```python
from build123d import *

# Parameters (mm, degrees)
SKETCH_1_W      = 292
SKETCH_1_H      = 160
SKETCH_1_R      = 1.5
SKETCH_1_W_2    = 60
SKETCH_1_H_2    = 80
EXTRUDE_1_DEPTH = 2


with BuildPart() as part:
    # 草图1 → 凸台-拉伸1 (new body)
    with BuildSketch(Plane(origin=(0, 0, 0), x_dir=(1, 0, 0), z_dir=(0, 1, 0))):
        with Locations((146, 80)):
            Rectangle(SKETCH_1_W, SKETCH_1_H)
        with Locations(Location((3, 140, 0), (0, 0, 270))):
            Circle(SKETCH_1_R, mode=Mode.SUBTRACT)
        with Locations(Location((3, 120, 0), (0, 0, 270))):
            Circle(SKETCH_1_R, mode=Mode.SUBTRACT)
        with Locations(Location((3, 40, 0), (0, 0, 270))):
            Circle(SKETCH_1_R, mode=Mode.SUBTRACT)
        with Locations(Location((3, 20, 0), (0, 0, 270))):
            Circle(SKETCH_1_R, mode=Mode.SUBTRACT)
        with Locations(Location((289, 20, 0), (0, 0, 90))):
            Circle(SKETCH_1_R, mode=Mode.SUBTRACT)
        with Locations(Location((289, 40, 0), (0, 0, 90))):
            Circle(SKETCH_1_R, mode=Mode.SUBTRACT)
        with Locations(Location((289, 120, 0), (0, 0, 90))):
            Circle(SKETCH_1_R, mode=Mode.SUBTRACT)
        with Locations(Location((289, 140, 0), (0, 0, 90))):
            Circle(SKETCH_1_R, mode=Mode.SUBTRACT)
        with Locations(Location((187, 120, 0), (0, 0, 270))):
            Circle(SKETCH_1_R, mode=Mode.SUBTRACT)
        with Locations(Location((262, 120, 0), (0, 0, 270))):
            Circle(SKETCH_1_R, mode=Mode.SUBTRACT)
        with Locations(Location((262, 98, 0), (0, 0, 270))):
            Circle(SKETCH_1_R, mode=Mode.SUBTRACT)
        with Locations(Location((187, 98, 0), (0, 0, 270))):
            Circle(SKETCH_1_R, mode=Mode.SUBTRACT)
        with Locations(Location((187, 105, 0), (0, 0, 270))):
            Circle(SKETCH_1_R, mode=Mode.SUBTRACT)
        with Locations(Location((262, 105, 0), (0, 0, 270))):
            Circle(SKETCH_1_R, mode=Mode.SUBTRACT)
        with Locations(Location((187, 83, 0), (0, 0, 270))):
            Circle(SKETCH_1_R, mode=Mode.SUBTRACT)
        with Locations(Location((262, 83, 0), (0, 0, 270))):
            Circle(SKETCH_1_R, mode=Mode.SUBTRACT)
        with Locations(Location((187, 90, 0), (0, 0, 270))):
            Circle(SKETCH_1_R, mode=Mode.SUBTRACT)
        with Locations(Location((262, 90, 0), (0, 0, 270))):
            Circle(SKETCH_1_R, mode=Mode.SUBTRACT)
        with Locations(Location((187, 68, 0), (0, 0, 270))):
            Circle(SKETCH_1_R, mode=Mode.SUBTRACT)
        with Locations(Location((262, 68, 0), (0, 0, 270))):
            Circle(SKETCH_1_R, mode=Mode.SUBTRACT)
        with Locations(Location((187, 75, 0), (0, 0, 270))):
            Circle(SKETCH_1_R, mode=Mode.SUBTRACT)
        with Locations(Location((262, 75, 0), (0, 0, 270))):
            Circle(SKETCH_1_R, mode=Mode.SUBTRACT)
        with Locations(Location((187, 53, 0), (0, 0, 270))):
            Circle(SKETCH_1_R, mode=Mode.SUBTRACT)
        with Locations(Location((262, 53, 0), (0, 0, 270))):
            Circle(SKETCH_1_R, mode=Mode.SUBTRACT)
        with Locations(Location((187, 60, 0), (0, 0, 270))):
            Circle(SKETCH_1_R, mode=Mode.SUBTRACT)
        with Locations(Location((262, 60, 0), (0, 0, 270))):
            Circle(SKETCH_1_R, mode=Mode.SUBTRACT)
        with Locations(Location((187, 38, 0), (0, 0, 270))):
            Circle(SKETCH_1_R, mode=Mode.SUBTRACT)
        with Locations(Location((262, 38, 0), (0, 0, 270))):
            Circle(SKETCH_1_R, mode=Mode.SUBTRACT)
        with Locations(Location((40, 145, 0), (0, 0, 270))):
            Circle(SKETCH_1_R, mode=Mode.SUBTRACT)
        with Locations(Location((80, 145, 0), (0, 0, 270))):
            Circle(SKETCH_1_R, mode=Mode.SUBTRACT)
        with Locations(Location((40, 15, 0), (0, 0, 270))):
            Circle(SKETCH_1_R, mode=Mode.SUBTRACT)
        with Locations(Location((80, 15, 0), (0, 0, 270))):
            Circle(SKETCH_1_R, mode=Mode.SUBTRACT)
        with Locations((60, 80)):
            Rectangle(SKETCH_1_W_2, SKETCH_1_H_2, mode=Mode.SUBTRACT)
        with BuildLine():
            Line((197, 124), (252, 124))
            ThreePointArc((252, 124), (256, 120), (252, 116))
            Line((252, 116), (197, 116))
            ThreePointArc((197, 116), (193, 120), (197, 124))
        make_face(mode=Mode.SUBTRACT)
        with BuildLine():
            Line((197, 101), (252, 101))
            ThreePointArc((252, 101), (256, 105), (252, 109))
            Line((252, 109), (197, 109))
            ThreePointArc((197, 109), (193, 105), (197, 101))
        make_face(mode=Mode.SUBTRACT)
        with BuildLine():
            Line((197, 86), (252, 86))
            ThreePointArc((252, 86), (256, 90), (252, 94))
            Line((252, 94), (197, 94))
            ThreePointArc((197, 94), (193, 90), (197, 86))
        make_face(mode=Mode.SUBTRACT)
        with BuildLine():
            Line((197, 71), (252, 71))
            ThreePointArc((252, 71), (256, 75), (252, 79))
            Line((252, 79), (197, 79))
            ThreePointArc((197, 79), (193, 75), (197, 71))
        make_face(mode=Mode.SUBTRACT)
        with BuildLine():
            Line((197, 56), (252, 56))
            ThreePointArc((252, 56), (256, 60), (252, 64))
            Line((252, 64), (197, 64))
            ThreePointArc((197, 64), (193, 60), (197, 56))
        make_face(mode=Mode.SUBTRACT)
        with BuildLine():
            Line((197, 49), (252, 49))
            ThreePointArc((252, 49), (256, 45), (252, 41))
            Line((252, 41), (197, 41))
            ThreePointArc((197, 41), (193, 45), (197, 49))
        make_face(mode=Mode.SUBTRACT)
        with BuildLine():
            Line((197, 34), (252, 34))
            ThreePointArc((252, 34), (256, 30), (252, 26))
            Line((252, 26), (197, 26))
            ThreePointArc((197, 26), (193, 30), (197, 34))
        make_face(mode=Mode.SUBTRACT)
        with BuildLine():
            Line((118.5, 116), (173.5, 116))
            ThreePointArc((173.5, 116), (177.5, 120), (173.5, 124))
            Line((173.5, 124), (118.5, 124))
            ThreePointArc((118.5, 124), (114.5, 120), (118.5, 116))
        make_face(mode=Mode.SUBTRACT)
        with BuildLine():
            Line((118.5, 109), (173.5, 109))
            ThreePointArc((173.5, 109), (177.5, 105), (173.5, 101))
            Line((173.5, 101), (118.5, 101))
            ThreePointArc((118.5, 101), (114.5, 105), (118.5, 109))
        make_face(mode=Mode.SUBTRACT)
        with BuildLine():
            Line((118.5, 94), (173.5, 94))
            ThreePointArc((173.5, 94), (177.5, 90), (173.5, 86))
            Line((173.5, 86), (118.5, 86))
            ThreePointArc((118.5, 86), (114.5, 90), (118.5, 94))
        make_face(mode=Mode.SUBTRACT)
        with BuildLine():
            Line((118.5, 79), (173.5, 79))
            ThreePointArc((173.5, 79), (177.5, 75), (173.5, 71))
            Line((173.5, 71), (118.5, 71))
            ThreePointArc((118.5, 71), (114.5, 75), (118.5, 79))
        make_face(mode=Mode.SUBTRACT)
        with BuildLine():
            Line((118.5, 64), (173.5, 64))
            ThreePointArc((173.5, 64), (177.5, 60), (173.5, 56))
            Line((173.5, 56), (118.5, 56))
            ThreePointArc((118.5, 56), (114.5, 60), (118.5, 64))
        make_face(mode=Mode.SUBTRACT)
        with BuildLine():
            Line((118.5, 49), (173.5, 49))
            ThreePointArc((173.5, 49), (177.5, 45), (173.5, 41))
            Line((173.5, 41), (118.5, 41))
            ThreePointArc((118.5, 41), (114.5, 45), (118.5, 49))
        make_face(mode=Mode.SUBTRACT)
        with BuildLine():
            Line((118.5, 34), (173.5, 34))
            ThreePointArc((173.5, 34), (177.5, 30), (173.5, 26))
            Line((173.5, 26), (118.5, 26))
            ThreePointArc((118.5, 26), (114.5, 30), (118.5, 34))
        make_face(mode=Mode.SUBTRACT)
    extrude(amount=EXTRUDE_1_DEPTH)


solid = part.part
```
Check sheet for the modelled part. Datum: model origin and axes. Units: mm. Coordinates: 2 decimals unless noted, no trailing zeros. Use a Markdown table: item, result.
1. Sectioned sample at A-A (y = 1.35). Give the number of separate pieces and of enclosed holes in the cut face, plus the area to 3 significant figures.
Reported:
| item | result |
|---|---|
| separate pieces | 1 |
| enclosed holes | 47 |
| area | 34,800 mm2 |
2. Go/stop test with a flat-tipped pin: pin 1 Ø1 at (x, y) = (211.5, 1) entering from +Z. Record where the tip stops, or that it passes through.
Reported:
| item | result |
|---|---|
| pin 1 | stops at z = 0 |
3. Scan lines: line 1 along X through (y, z) = (0.75, -15); line 2 along X through (y, z) = (1.15, -140); line 3 along Z through (x, y) = (289, 0.6). Record each from-to range of solid material in increasing order.
Reported:
| item | result |
|---|---|
| line 1 | x = 0 to 38.5, 41.5 to 78.5, 81.5 to 292 |
| line 2 | x = 0 to 1.5, 4.5 to 287.5, 290.5 to 292 |
| line 3 | z = -160 to -141.5, -138.5 to -121.5, -118.5 to -41.5, -38.5 to -21.5, -18.5 to 0 |
4. Release check for a two-part mould opening along Y. For faces 1 (the flat face through (144, 2, -81)), 2 (the flat face through (144, 0, -81)) record: pulls with the +Y half, pulls with the -Y half, needs draft (parallel to the pull), parting line crosses it, or undercut.
Reported:
| item | result |
|---|---|
| face 1 | pulls with the +Y half |
| face 2 | pulls with the -Y half |
